```python
from build123d import *

# Parameters (mm, degrees)
SKETCH1_R           = 125
SKETCH1_R_2         = 1.55
SKETCH1_R_3         = 32.5
BOSS_EXTRUDE1_DEPTH = 1.5
SKETCH2_R           = 1.549999995
SKETCH2_R_2         = 1.550000001
SKETCH2_R_3         = 1.550000005
SKETCH2_R_4         = 1.55
CUT_EXTRUDE1_DEPTH  = 1.5
SKETCH3_R           = 1.55
CUT_EXTRUDE2_DEPTH  = 1.5


with BuildPart() as part:
    # Sketch1 → Boss-Extrude1 (new body)
    with BuildSketch(Plane(origin=(0, 0, 0), x_dir=(1, 0, 0), z_dir=(0, 1, 0))):
        Circle(SKETCH1_R)
        with Locations((0, -37.5)):
            Circle(SKETCH1_R_2, mode=Mode.SUBTRACT)
        with Locations((0, 37.5)):
            Circle(SKETCH1_R_2, mode=Mode.SUBTRACT)
        with Locations((37.5, 0)):
            Circle(SKETCH1_R_2, mode=Mode.SUBTRACT)
        with Locations((-37.5, 0)):
            Circle(SKETCH1_R_2, mode=Mode.SUBTRACT)
        Circle(SKETCH1_R_3, mode=Mode.SUBTRACT)
    extrude(amount=BOSS_EXTRUDE1_DEPTH)

    # Sketch2 → Cut-Extrude1 (cut)
    with BuildSketch(Plane(origin=(0, 1.5, 0), x_dir=(1, 0, 0), z_dir=(0, 1, 0))):
        with Locations((-71.269065604, 92.835829434)):
            Circle(SKETCH2_R)
        with Locations((-35.913726545, 57.480490375)):
            Circle(SKETCH2_R)
        with Locations((-92.835822431, 71.269072608)):
            Circle(SKETCH2_R)
        with Locations((-57.480483371, 35.913733548)):
            Circle(SKETCH2_R)
        with Locations((71.269072585, 92.835822411)):
            Circle(SKETCH2_R_2)
        with Locations((92.835829411, 71.269065585)):
            Circle(SKETCH2_R_2)
        with Locations((35.913733525, 57.480483351)):
            Circle(SKETCH2_R_2)
        with Locations((57.480490352, 35.913726525)):
            Circle(SKETCH2_R_2)
        with Locations((92.835822388, -71.269072605)):
            Circle(SKETCH2_R_3)
        with Locations((71.269065562, -92.835829431)):
            Circle(SKETCH2_R_3)
        with Locations((57.480483329, -35.913733545)):
            Circle(SKETCH2_R_3)
        with Locations((35.913726502, -57.480490371)):
            Circle(SKETCH2_R_3)
        with Locations((-71.269072628, -92.835822408)):
            Circle(SKETCH2_R_2)
        with Locations((-92.835829454, -71.269065582)):
            Circle(SKETCH2_R_2)
        with Locations((-35.913733568, -57.480483348)):
            Circle(SKETCH2_R_2)
        with Locations((-57.480490394, -35.913726522)):
            Circle(SKETCH2_R_2)
        with Locations((-57.480490394, -79.047240175)):
            Circle(SKETCH2_R_4)
        with Locations((-79.047247221, -57.480483348)):
            Circle(SKETCH2_R_4)
    extrude(amount=-CUT_EXTRUDE1_DEPTH, mode=Mode.SUBTRACT)

    # Sketch3 → Cut-Extrude2 (cut)
    with BuildSketch(Plane(origin=(0, 1.5, 0), x_dir=(1, 0, 0), z_dir=(0, 1, 0))):
        with Locations((-100, 15)):
            Circle(SKETCH3_R)
        with Locations((-100, -15)):
            Circle(SKETCH3_R)
        with Locations((-85, 0)):
            Circle(SKETCH3_R)
        with Locations((-115, 0)):
            Circle(SKETCH3_R)
    extrude(amount=-CUT_EXTRUDE2_DEPTH, mode=Mode.SUBTRACT)


solid = part.part
```
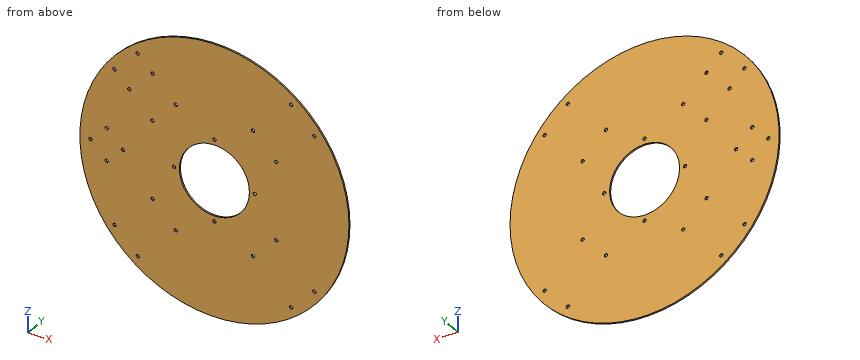
Read the model definition and answer for the solid it produces. Units are mm, in the model's axes. Round coordinates to 2 decimals unless told otherwise and drop trailing zeros. Write each loop counter-clockwise with the first axis right and the second up, starting at its lowest first coordinate (ties: lowest second). Pieces come first, ordered by that corner, then holes. Notation, with made-up numbers: (77, -31) -> (102, -31) arc R5 cw to (102, -27) -> close; hole circle Ø11 at (19.25, 34). An arc over 180 degrees is marked (long way). Answer in a Markdown table with one row per item. Add a question column.
1) Find section B-B, the plane x = -18.5. Determine the outline of the cut face in (y, z).
2) Find section D-D, the plane z = -79.5. Determine the outline of the cut face in (x, y), and give its area (3 significant figures).
3) Consider line 1 (X direction, y = 0.4, z = -38.5); line 2 (X direction, y = 0.3, z = 26.5). Determine where each line is inside the solid, lowest interval first.
4) Find section A-A, the plane y = 0.3. State how many separate pieces and enclosed holes the cut face has, and give its area (3 significant figures).
5) Find section C-C, the plane x = 82. Determine the outline of the cut face in (y, z), and give its area (3 significant figures).
Findings below:
| question | item | result |
|---|---|---|
| 1 | outline | (0, -123.62) -> (1.5, -123.62) -> (1.5, -26.72) -> (0, -26.72) -> close; (0, 26.72) -> (1.5, 26.72) -> (1.5, 123.62) -> (0, 123.62) -> close |
| 2 | outline | (-96.46, 0) -> (96.46, 0) -> (96.46, 1.5) -> (-96.46, 1.5) -> close |
| 2 | area | 289 mm² |
| 3 | line 1 | -118.92 to -1.18, 1.18 to 118.92 |
| 3 | line 2 | -122.16 to -18.81, 18.81 to 122.16 |
| 4 | separate pieces | 1 |
| 4 | enclosed holes | 27 |
| 4 | area | 45,600 mm² |
| 5 | outline | (0, -94.35) -> (1.5, -94.35) -> (1.5, 94.35) -> (0, 94.35) -> close |
| 5 | area | 283 mm² |
